from build123d import *

# Parameters (mm, degrees)
F0_W     = 100
F0_H     = 50
F1_DEPTH = 40
F2_W     = 46.505556
F2_H     = 30.397546
F3_DEPTH = 99
F4_R     = 5


with BuildPart() as f1:
    # F0 (on Top) → F1 (new body)
    with BuildSketch(Plane.XY):
        Rectangle(F0_W, F0_H)
    extrude(amount=F1_DEPTH)

    # F2 (on face) → F3 (cut)
    with BuildSketch(Plane.XZ.offset(25)):
        with Locations((18.68185, 39.786866)):
            Rectangle(F2_W, F2_H)
    extrude(amount=-F3_DEPTH, mode=Mode.SUBTRACT)

    # F4
    f4_edges = [f1.edges().sort_by_distance(p)[0] for p in [
        (-4.570928, 0, 24.588093),
        (41.934628, 0, 24.588093),
    ]]
    fillet(f4_edges, radius=F4_R)


solid = f1.part
Read the model definition and answer for the solid it produces. Units are mm, in the model's axes. A direction names the side the tool comes from. Coordinates: 2 decimals unless noted, no trailing zeros. Loops run counter-clockwise (first coordinate to the right, second up) from the corner with the lowest first, then second, coordinate; pieces in that order, holes last. Notation, with made-up numbers: (19.5, 46.25) -> (71.5, 46.25) arc R21 ccw to (71.5, 58.25) -> close; hole circle Ø9 at (-29.75, 66). An arc over 180 degrees is marked (long way). Answer in a Markdown table with one row per item.
Item 1: A cutting plane is placed at B-B on y = -3.5. Determine the outline of the cut face in (x, z).
Returned:
| item | result |
|---|---|
| outline | (-50, 0) -> (50, 0) -> (50, 40) -> (41.93, 40) -> (41.93, 29.59) arc R5 cw to (36.93, 24.59) -> (0.43, 24.59) arc R5 cw to (-4.57, 29.59) -> (-4.57, 40) -> (-50, 40) -> close |
Item 2: For faces 5 (the flat face through (41.935, 0, 35)), 6 (the flat face through (46, 0, 40)), determine the directions among +Z, -Z, +X, -X, +Y, -Y from which every point of the face is accessible in a straight line to the end or side of a thin tool.
Returned:
| item | result |
|---|---|
| face 5 | +Z, +Y, -Y |
| face 6 | +Z, +X, -X, +Y, -Y |
Item 3: A cutting plane is placed at C-C on z = 28. Determine the outline of the cut face in (x, y).
Returned:
| item | result |
|---|---|
| outline | (-50, -25) -> (-4.31, -25) -> (-4.31, 25) -> (-50, 25) -> close; (41.68, -25) -> (50, -25) -> (50, 25) -> (41.68, 25) -> close |
Item 4: For a pull along X with two mould halves and no side action, classify faces 1 (the flat face through (-50, 0, 20)), 2 (the flat face through (-28, 0, 40)), 3 (the flat face through (50, 0, 20)), 4 (the flat face through (-4.571, 0, 35)) as released by +X, released by -X, zero draft, split by the parting line, or undercut.
Returned:
| item | result |
|---|---|
| face 1 | released by -X |
| face 2 | zero draft |
| face 3 | released by +X |
| face 4 | undercut |
Item 5: A cutting plane is placed at A-A on z = 37. Determine the outline of the cut face in (x, y), plus the area to 3 significant figures.
Returned:
| item | result |
|---|---|
| outline | (-50, -25) -> (-4.57, -25) -> (-4.57, 25) -> (-50, 25) -> close; (41.93, -25) -> (50, -25) -> (50, 25) -> (41.93, 25) -> close |
| area | 2,670 mm^2 |
Item 6: Straight lines are drawn through the part: line 1 along X through (y, z) = (16, 34.5); line 2 along Z through (x, y) = (6, -20); line 3 along X through (y, z) = (-16, 28). For each, find the intervals that lie inside material, in ascending order. Write a range as [from, to].
Returned:
| item | result |
|---|---|
| line 1 | x = [-50, -4.57], [41.93, 50] |
| line 2 | z = [0, 24.59] |
| line 3 | x = [-50, -4.31], [41.68, 50] |
Item 7: A cutting plane is placed at D-D on x = 35.5. Determine the outline of the cut face in (y, z).
Returned:
| item | result |
|---|---|
| outline | (-25, 0) -> (25, 0) -> (25, 24.59) -> (-25, 24.59) -> close |
Item 8: This flat-tipped pin is pushed along its axis until it touches: P1, Ø5, axis at x = 1, y = 4, coming from the -Z side. Where does it stop, or does it pass through?
Returned:
| item | result |
|---|---|
| P1 | stops at z = 0 |
